```python
from build123d import *

# Parameters (mm, degrees)
F1_DEPTH = 15
F2_DEPTH = 4
F4_DEPTH = 250
F6_DEPTH = 7


with BuildPart() as f1:
    # F0 (on Top) → F1 (new body)
    with BuildSketch(Plane.XY):
        with BuildLine():
            ThreePointArc((-76.5, -11.9921219791), (0, 0), (76.5, -11.9921219791))
            Line((76.5, -11.9921219791), (82.8024758084, -11.9921219791))
            ThreePointArc((82.8024758084, -11.9921219791), (0, 2), (-82.8024758084, -11.9921219791))
            Line((-82.8024758084, -11.9921219791), (-76.5, -11.9921219791))
        make_face()
    extrude(amount=F1_DEPTH)

    # F2 (add): faces of the model
    f2_faces = [f1.faces().sort_by_distance(p)[0] for p in [
        (-79.6512379042, -11.9921219791, 7.5),
        (79.6512379042, -11.9921219791, 7.5),
    ]]
    extrude(f2_faces, amount=F2_DEPTH)

    # F3 (on face) → F4 (cut)
    with BuildSketch(Plane.YZ.offset(82.8024758084)):
        Polygon((-11.9921219791, 0), (-15.9921219791, 15), (-15.9921219791, 0), align=None)
    extrude(amount=-F4_DEPTH, mode=Mode.SUBTRACT)

    # F5 (on face) → F6 (join)
    with BuildSketch(Plane(origin=(0, -11.1959645033, -2.9855905342), x_dir=(1, 0, 0), z_dir=(0, -0.9662349396, -0.2576626506))):
        with BuildLine():
            ThreePointArc((-80.6512379042, 9.9700432719), (-80.2636103399, 7.4827028894), (-78.1512379042, 8.8520092831))
            ThreePointArc((-78.1512379042, 8.8520092831), (-78.2819315104, 9.4643817188), (-78.6512379042, 9.9700432719))
            ThreePointArc((-78.6512379042, 9.9700432719), (-79.6512379042, 10.3520092831), (-80.6512379042, 9.9700432719))
        make_face()
        with BuildLine():
            ThreePointArc((-80.6512379042, 9.9700432719), (-79.6512379042, 10.3520092831), (-78.6512379042, 9.9700432719))
            Line((-78.6512379042, 9.9700432719), (-78.6512379042, 11.7339752944))
            ThreePointArc((-78.6512379042, 11.7339752944), (-79.6512379042, 11.3520092831), (-80.6512379042, 11.7339752944))
            Line((-80.6512379042, 11.7339752944), (-80.6512379042, 9.9700432719))
        make_face()
        with BuildLine():
            ThreePointArc((-80.6512379042, 11.7339752944), (-79.6512379042, 11.3520092831), (-78.6512379042, 11.7339752944))
            ThreePointArc((-78.6512379042, 11.7339752944), (-78.2819315104, 12.2396368474), (-78.1512379042, 12.8520092831))
            ThreePointArc((-78.1512379042, 12.8520092831), (-80.2636103399, 14.2213156769), (-80.6512379042, 11.7339752944))
        make_face()
        with BuildLine():
            ThreePointArc((80.6512379042, 9.9700432719), (79.6512379042, 10.3520092831), (78.6512379042, 9.9700432719))
            ThreePointArc((78.6512379042, 9.9700432719), (79.0388654685, 7.4827028894), (81.1512379042, 8.8520092831))
            ThreePointArc((81.1512379042, 8.8520092831), (81.020544298, 9.4643817188), (80.6512379042, 9.9700432719))
        make_face()
        with BuildLine():
            Line((78.6512379042, 11.7339752944), (78.6512379042, 9.9700432719))
            ThreePointArc((78.6512379042, 9.9700432719), (79.6512379042, 10.3520092831), (80.6512379042, 9.9700432719))
            Line((80.6512379042, 9.9700432719), (80.6512379042, 11.7339752944))
            ThreePointArc((80.6512379042, 11.7339752944), (79.6512379042, 11.3520092831), (78.6512379042, 11.7339752944))
        make_face()
        with BuildLine():
            ThreePointArc((81.1512379042, 12.8520092831), (79.0388654685, 14.2213156769), (78.6512379042, 11.7339752944))
            ThreePointArc((78.6512379042, 11.7339752944), (79.6512379042, 11.3520092831), (80.6512379042, 11.7339752944))
            ThreePointArc((80.6512379042, 11.7339752944), (81.020544298, 12.2396368474), (81.1512379042, 12.8520092831))
        make_face()
    extrude(amount=F6_DEPTH)


solid = f1.part
```
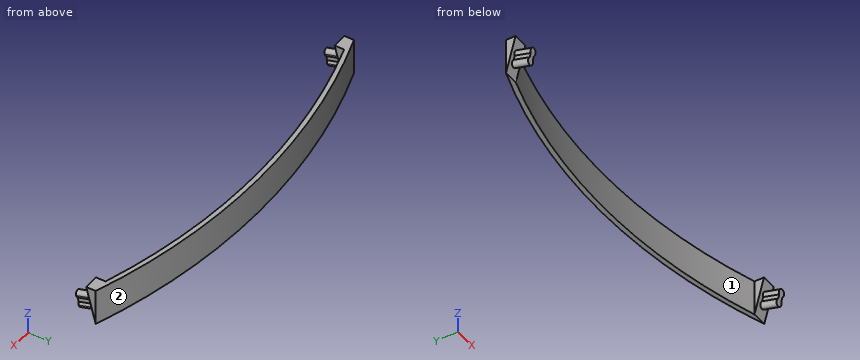
Check sheet for the modelled part. Datum: model origin and axes. Units: mm. Face numbers are marked on the shaded views. Give positions to 0.01 mm unless a question says otherwise; leave off trailing zeros. Order: outer loops, then holes, each group sorted by start corner. A loop starts at its lowest first (then second) coordinate and runs counter-clockwise, first axis right, second up. Notation, with made-up numbers: M 32,23.5 L 50,23.5 A18 ccw 50,29.5 Z; hole C 28.5,70.5 d3. An arc over 180 degrees is marked long. Answer in a Markdown table with one row per item. Add a question column.
Q1. Gauge pin test, flat ends, axial feed: pin 1 Ø3 at (y, z) = (-17.5, 7) entering from +X; pin 2 Ø6 at (x, z) = (62, 3.5) entering from -Y; pin 3 Ø1.5 at (x, z) = (10.5, 9.5) entering from +Y; pin 4 Ø10 at (x, y) = (9, -10) entering from -Z. Record the tip position at first contact, or that the pin passes through.
Q2. Sectioned sample at B-B, the plane z = 13.25. Record the boundary of the cut face in (x, y).
Q3. Sectioned sample at A-A, the plane y = -7.75. Record the boundary of the cut face in (x, z), and give its area (3 significant figures).
Q4. Release check for a two-part mould opening along X. For the marked faces 1 and 2 record: released by +X, released by -X, zero draft, split by the parting line, or undercut.
Q5. Sectioned sample at C-C, the plane x = -50. Record the boundary of the cut face in (y, z).
Q6. Sectioned sample at D-D, the plane x = -4. Record the boundary of the cut face in (y, z).
Q7. Thickness scan on L1, parallel to X at y = -13, z = 14.5; L2, parallel to X at y = -16, z = 6; L3, parallel to Y at x = 66.5, z = 3.25. Record the ranges inside material, lowest first.
Verdict:
| question | item | result |
|---|---|---|
| 1 | pin 1 | x = 81.15 |
| 1 | pin 2 | y = -8.6 |
| 1 | pin 3 | y = 1.81 |
| 1 | pin 4 | through |
| 2 | outline | M -82.8,-15.53 L -76.5,-15.53 L -76.5,-11.99 A250 cw 76.5,-11.99 L 76.5,-15.53 L 82.8,-15.53 L 82.8,-11.99 A252 ccw -82.8,-11.99 Z |
| 3 | outline | M -69.42,0 L -61.77,0 L -61.77,15 L -69.42,15 Z; M 61.77,0 L 69.42,0 L 69.42,15 L 61.77,15 Z |
| 3 | area | 230 mm² |
| 4 | face 1 | undercut |
| 4 | face 2 | split by the parting line |
| 5 | outline | M -5.05,0 L -3.01,0 L -3.01,15 L -5.05,15 Z |
| 6 | outline | M -0.03,0 L 1.97,0 L 1.97,15 L -0.03,15 Z |
| 7 | L1 | -82.8 to -76.5, 76.5 to 82.8 |
| 7 | L2 | -80.7 to -78.6, 78.6 to 80.7 |
| 7 | L3 | -9.01 to -6.93 |
